Source: three-view drawing plus pictorial views. Frame: mm from the lowest corner of the part. A direction names the side the tool comes from. Give positions to 0.01 mm unless a question says otherwise; leave off trailing zeros. Loops run counter-clockwise (first coordinate to the right, second up) from the corner with the lowest first, then second, coordinate; pieces in that order, holes last. Notation, with made-up numbers: (57.25, 58.25) - (97.25, 58.25) arc R20 ccw to (97.25, 88.25) - close; hole circle Ø8 at (72.25, 88.25). An arc over 180 degrees is marked (long way). Answer in a Markdown table with one row per item.
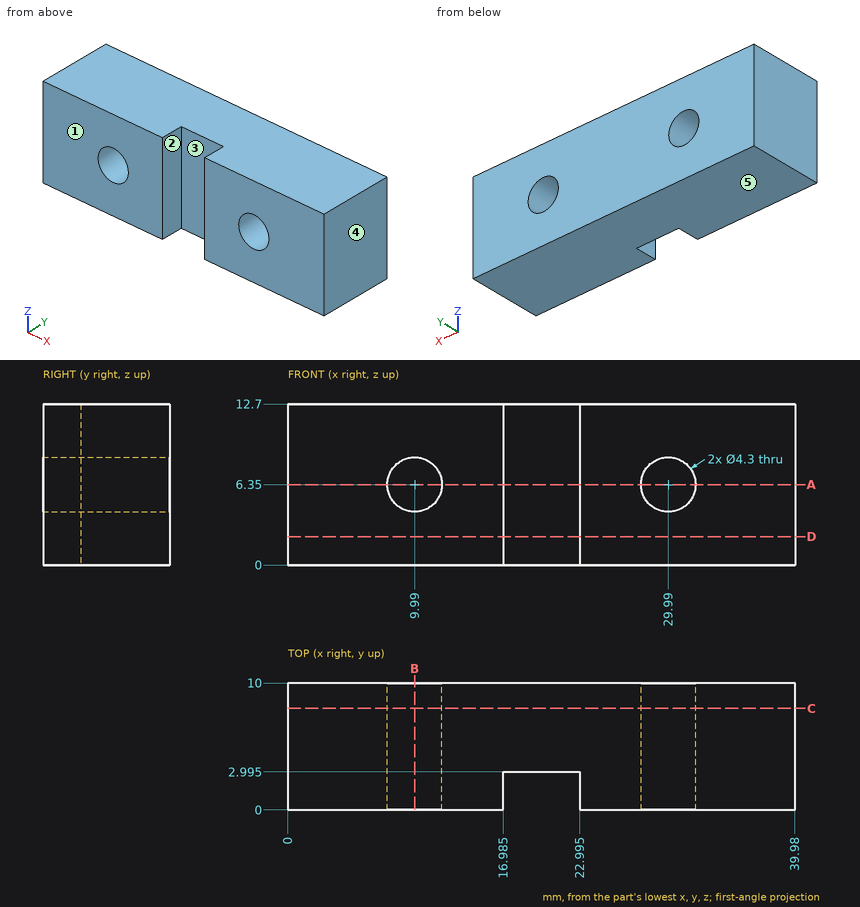
Q1. Draft query along X for the marked faces 3, 4 and 5. Return one class per face: pulls with the +X half, pulls with the -X half, needs draft (parallel to the pull), parting line crosses it, or undercut.
Check values:
| item | result |
|---|---|
| face 3 | undercut |
| face 4 | pulls with the +X half |
| face 5 | needs draft |
Q2. Cut plane B-B (x = 9.99). Output: boundary loops of the cut face in (y, z).
Check values:
| item | result |
|---|---|
| outline | (0, 0) - (10, 0) - (10, 4.2) - (0, 4.2) - close; (0, 8.5) - (10, 8.5) - (10, 12.7) - (0, 12.7) - close |
Q3. Material intervals for line 1 along X through (y, z) = (3.25, 6.35); line 2 along X through (y, z) = (0.5, 9.5) (3 decimals); line 3 along X through (y, z) = (1.5, 7) (3 decimals), sorted ascending.
Check values:
| item | result |
|---|---|
| line 1 | 0 to 7.84, 12.14 to 27.84, 32.14 to 39.98 |
| line 2 | 0 to 16.985, 22.995 to 39.98 |
| line 3 | 0 to 7.941, 12.039 to 16.985, 22.995 to 27.941, 32.039 to 39.98 |
Q4. Reachability of the marked faces 1 and 2 from +Z, -Z, +X, -X, +Y, -Y: full face, straight path, thin tool, end or side. Return the list, or none.
Check values:
| item | result |
|---|---|
| face 1 | +Z, -Z, +X, -X, -Y |
| face 2 | +Z, -Z, -Y |
Q5. Cut plane D-D (z = 2.25). Output: boundary loops of the cut face in (x, y) (3 decimals).
Check values:
| item | result |
|---|---|
| outline | (0, 0) - (16.985, 0) - (16.985, 2.995) - (22.995, 2.995) - (22.995, 0) - (39.98, 0) - (39.98, 10) - (0, 10) - close |
Q6. Cut plane A-A (z = 6.35). Output: boundary loops of the cut face in (x, y) (3 decimals), and give its area (3 significant figures).
Check values:
| item | result |
|---|---|
| outline | (0, 0) - (7.84, 0) - (7.84, 10) - (0, 10) - close; (12.14, 0) - (16.985, 0) - (16.985, 2.995) - (22.995, 2.995) - (22.995, 0) - (27.84, 0) - (27.84, 10) - (12.14, 10) - close; (32.14, 0) - (39.98, 0) - (39.98, 10) - (32.14, 10) - close |
| area | 296 mm² |
Q7. Cut plane C-C (y = 8). Output: boundary loops of the cut face in (x, z).
Check values:
| item | result |
|---|---|
| outline | (0, 0) - (39.98, 0) - (39.98, 12.7) - (0, 12.7) - close; hole circle Ø4.3 at (9.99, 6.35); hole circle Ø4.3 at (29.99, 6.35) |
